Here's how the part is built. I have some questions about the finished solid (model axes, mm). Face numbers are marked on the shaded views. Coordinates: 2 decimals unless noted, no trailing zeros. Loops run counter-clockwise (first coordinate to the right, second up) from the corner with the lowest first, then second, coordinate; pieces in that order, holes last.
```python
from build123d import *

# Parameters (mm, degrees)
ESQUISSE1_W             = 50
ESQUISSE1_H             = 35
BOSS_EXTRU_1_DEPTH      = 10
ESQUISSE2_R             = 5
ENL_V_MAT_EXTRU_1_DEPTH = 5
ESQUISSE3_R             = 1.375
ESQUISSE3_R_2           = 3.5
ENL_V_MAT_EXTRU_2_DEPTH = 15
ESQUISSE4_R             = 11
ENL_V_MAT_EXTRU_3_DEPTH = 2.5
ESQUISSE5_R             = 2.25
ENL_V_MAT_EXTRU_4_DEPTH = 2.5
ESQUISSE6_R             = 2
ENL_V_MAT_EXTRU_5_DEPTH = 10


with BuildPart() as part:
    # Esquisse1 → Boss.-Extru.1 (new body)
    with BuildSketch(Plane(origin=(0, 0, 0), x_dir=(1, 0, 0), z_dir=(0, 1, 0))):
        Rectangle(ESQUISSE1_W, ESQUISSE1_H)
    extrude(amount=BOSS_EXTRU_1_DEPTH)

    # Esquisse2 → Enlèv. mat.-Extru.1 (cut)
    with BuildSketch(Plane(origin=(0, 10, 0), x_dir=(1, 0, 0), z_dir=(0, 1, 0))):
        with Locations(Location((0, 2.5, 0), (0, 0, 270))):
            Circle(ESQUISSE2_R)
    extrude(amount=-ENL_V_MAT_EXTRU_1_DEPTH, mode=Mode.SUBTRACT)

    # Esquisse3 → Enlèv. mat.-Extru.2 (cut)
    with BuildSketch(Plane(origin=(0, 10, 0), x_dir=(1, 0, 0), z_dir=(0, 1, 0))):
        with Locations(Location((-1.811733316, 9.261480784, 0), (0, 0, 270))):
            Circle(ESQUISSE3_R)
        with Locations(Location((6.761480784, 0.688266684, 0), (0, 0, 270))):
            Circle(ESQUISSE3_R)
        with Locations(Location((-4.949747468, -2.449747468, 0), (0, 0, 270))):
            Circle(ESQUISSE3_R)
        with Locations(Location((0, 2.5, 0), (0, 0, 270))):
            Circle(ESQUISSE3_R_2)
    extrude(amount=-ENL_V_MAT_EXTRU_2_DEPTH, mode=Mode.SUBTRACT)

    # Esquisse4 → Enlèv. mat.-Extru.3 (cut)
    with BuildSketch(Plane(origin=(0, 10, 0), x_dir=(1, 0, 0), z_dir=(0, 1, 0))):
        with Locations(Location((0, 2.5, 0), (0, 0, 270))):
            Circle(ESQUISSE4_R)
    extrude(amount=-ENL_V_MAT_EXTRU_3_DEPTH, mode=Mode.SUBTRACT)

    # Esquisse5 → Enlèv. mat.-Extru.4 (cut)
    with BuildSketch(Plane.XZ):
        with Locations(Location((-4.949747468, 2.449747468, 0), (0, 0, 270))):
            Circle(ESQUISSE5_R)
        with Locations(Location((6.761480784, -0.688266684, 0), (0, 0, 270))):
            Circle(ESQUISSE5_R)
        with Locations(Location((-1.811733316, -9.261480784, 0), (0, 0, 270))):
            Circle(ESQUISSE5_R)
    extrude(amount=-ENL_V_MAT_EXTRU_4_DEPTH, mode=Mode.SUBTRACT)

    # Esquisse6 → Enlèv. mat.-Extru.5 (cut)
    with BuildSketch(Plane.XY.offset(17.5)):
        with Locations((-20, 5)):
            Circle(ESQUISSE6_R)
        with Locations((20, 5)):
            Circle(ESQUISSE6_R)
    extrude(amount=-ENL_V_MAT_EXTRU_5_DEPTH, mode=Mode.SUBTRACT)


solid = part.part
```
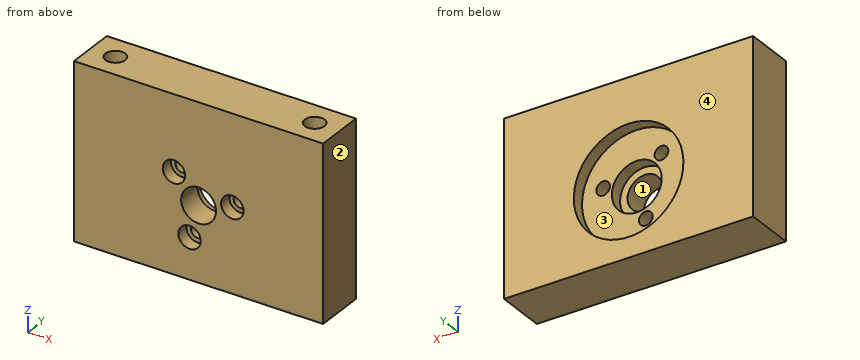
1. For pin 1 (2.5 mm diameter, centred on x = 20, y = 5, fed in from +Z); pin 2 (1.3 mm diameter, centred on x = -4, z = 2, fed in from -Y); pin 3 (7 mm diameter, centred on x = 6.76, z = -0.69, fed in from +Y), each with a flat end and sliding along its axis, tell me the tip position at first contact or that it passes through.
2. We'd pull the mould along X, two halves only. Please class the marked faces 1, 2, 3 and 4: +X half, -X half, draft (parallel to the pull), parting line (faces both ways), or undercut.
3. I need wall thicknesses on line 1 along Z through (x, y) = (-2.5, 0.5); line 2 along X through (y, z) = (5.6, -2.5); line 3 along X through (y, z) = (4.75, 11). Which ranges of each line are inside material? Lowest first, please.
4. I want a section at D-D (z = 10.5). Please give me the cut outline in (x, y), then the cut area to 3 significant figures.
5. I want a section at C-C (y = 1.5). Please give me the cut outline in (x, z), then the cut area to 3 significant figures.
6. I want a section at A-A (x = 20). Please give me the cut outline in (y, z), then the cut area to 3 significant figures.
7. I want a section at B-B (z = -4.5). Please give me the cut outline in (x, y), then the cut area to 3 significant figures.
Response values:
1. pin 1: stops at z = 7.5
1. pin 2: stops at y = 2.5
1. pin 3: stops at y = 7.5
2. face 1: undercut
2. face 2: +X half
2. face 3: undercut
2. face 4: draft
3. line 1: z = -17.5 to -11.4, -7.12 to -4.95, -0.05 to 17.5
3. line 2: x = -25 to -5, 5 to 25
3. line 3: x = -25 to -21.98, -18.02 to 18.02, 21.98 to 25
4. outline: (-25, 0) - (25, 0) - (25, 10) - (-25, 10) - close; hole circle Ø4 at (-20, 5); hole circle Ø4 at (20, 5)
4. area: 475 mm2
5. outline: (-25, -17.5) - (25, -17.5) - (25, 17.5) - (-25, 17.5) - close; hole circle Ø4.5 at (-4.95, 2.45); hole circle Ø4.5 at (-1.81, -9.26); hole circle Ø7 at (0, -2.5); hole circle Ø4.5 at (6.76, -0.69)
5. area: 1,660 mm2
6. outline: (0, -17.5) - (10, -17.5) - (10, 17.5) - (7, 17.5) - (7, 7.5) - (3, 7.5) - (3, 17.5) - (0, 17.5) - close
6. area: 310 mm2
7. outline: (-25, 0) - (-2.87, 0) - (-2.87, 5) - (-4.58, 5) - (-4.58, 7.5) - (-10.82, 7.5) - (-10.82, 10) - (-25, 10) - close; (2.87, 0) - (25, 0) - (25, 10) - (10.82, 10) - (10.82, 7.5) - (4.58, 7.5) - (4.58, 5) - (2.87, 5) - close
7. area: 394 mm2
